Autodesk Inventor part; units mm, degrees
ref_plane "YZ Plane" through (0, 0, 0) normal (1, 0, 0) x (0, 1, 0)
ref_plane "XZ Plane" through (0, 0, 0) normal (0, 1, 0) x (-1, 0, 0)
ref_plane "XY Plane" through (0, 0, 0) normal (0, 0, 1) x (1, 0, 0)
sketch "Szkic1" plane through (0, 0, 0) normal (0, 1, 0) x (-1, 0, 0)
  line L0 (0, 0) -> (-100, 0)
  line L1 (-100, 0) -> (-100, -14)
  line L2 (-100, -14) -> (0, -14)
  line L3 (0, -14) -> (0, 0)
  dimension "d0" = 100
  dimension "d1" = 14
extrude "Wyciągnięcie proste1" add sketch "Szkic1" along normal blind 0.5
sketch "Szkic2" plane through (0, 0.5, 0) normal (0, 1, 0) x (1, 0, 0)
  line L0 (100, 14) -> (0, 14)
  line L1 (80, 14) -> (20, 14)
  line L2 (20, 14) -> (20, 25)
  line L3 (20, 25) -> (80, 25)
  line L4 (80, 25) -> (80, 14)
  point P0 (0, 0)
  point P1 (50, 14)
  point P2 (50, 14)
  point P3 (50, 14)
  dimension "d4" = 60
  dimension "d5" = 11
extrude "Wyciągnięcie proste2" add sketch "Szkic2" against normal blind 0.5
sketch "Szkic3" plane through (80, 0.5, -14) normal (1, 0, 0) x (0, 0, -1)
  line L0 (0, 0) -> (11, 0)
  line L1 (0, -0.5) -> (0, 0)
  line L2 (11, -0.5) -> (0, -0.5)
  line L3 (11, 0) -> (11, -0.5)
  line L4 (11, 0) -> (23.4078, -2.7462)
  line L5 (11, -0.5) -> (23.3023, -3.2228)
  line L6 (23.3023, -3.2228) -> (23.4078, -2.7462)
  point P0 (-14, -0.5)
  dimension "d8" = 167.52
  dimension "d9" = 12.6
extrude "Wyciągnięcie proste3" add sketch "Szkic3" against normal up to surface (60 mm away) contours L4 L6 L5 L3
sketch "Szkic4" plane through (20, 0, -14) normal (-1, 0, 0) x (0, 0, 1)
  line L0 (-11, 0.5) -> (0, 0.5)
  line L1 (0, 0) -> (-11, 0)
  line L2 (0, 0.5) -> (14, 0.5)
  line L3 (0, 0) -> (14, 0)
  line L4 (0, 0) -> (14, 0)
  line L5 (14, 0) -> (14, 0.5)
  line L6 (0, 0.5) -> (14, 0.5)
  line L7 (0, 0) -> (0, 0.5)
  line L8 (-11, 0.5) -> (0, 0.5)
  line L9 (-23.4078, -2.2462) -> (-11, 0.5)
  line L10 (-23.3023, -2.7228) -> (-23.4078, -2.2462)
  line L11 (-11, 0) -> (-23.3023, -2.7228)
  line L12 (0, 0) -> (-11, 0)
  line L13 (0, 0.5) -> (0, 0)
  line L14 (-11, 0) -> (-23.3023, -2.7228)
  line L15 (-11, 0) -> (-11.1055, 0.4767)
extrude "Wyciągnięcie proste4" cut sketch "Szkic4" along normal through all both and the other way through all contours L0 L7 L1 L15 L9 | L2 L5 L3 L7
sketch "Szkic5" plane through (20, -2.7228, -37.3023) normal (-1, 0, 0) x (0, 0.2161, 0.9764)
  line L0 (15.5701, -17.2757) -> (12.57, -20.2756)
  line L1 (15.5701, -17.2757) -> (15.5704, -10.8597)
  line L2 (15.5708, -3.4757) -> (15.5704, -10.8597)
  point P0 (37.0093, -5.4025)
properties part number "tyl" material "Stal miękka, spawana"
Verification items for the finished model (mm, model axes). Give positions to 0.01 mm unless a question says otherwise; leave off trailing zeros. Loops run counter-clockwise (first coordinate to the right, second up) from the corner with the lowest first, then second, coordinate; pieces in that order, holes last.
1. Cross-section at B-B on y = -1.15. Record the cut outline in (x, z), and give its area (3 significant figures).
Derived:
outline: (20, -32.45) - (80, -32.45) - (80, -30.2) - (20, -30.2) - close
area: 136 mm2
2. Go/stop test with flat-tipped pins: P1, Ø1, axis at y = 0, z = -35.5, coming from the +X side; P2, Ø4, axis at x = 68, z = -27.5, coming from the +Y side; P3, Ø5, axis at x = 54, z = -30.5, coming from the -Y side. Record where each tip stops, or that it passes through.
Derived:
P1: passes through
P2: stops at y = 0.39
P3: stops at y = -1.77
3. Cross-section at A-A on x = 56. Record the cut outline in (y, z).
Derived:
outline: (-2.72, -37.3) - (-2.25, -37.41) - (0.48, -25.11) - (0, -25) - close
4. Material ranges on probe 1 along Y at (x, z) = (70.5, -35); probe 2 along Y at (x, z) = (77, -31.5), recorded low to high.
Derived:
probe 1: y = -2.21 to -1.71
probe 2: y = -1.44 to -0.94
